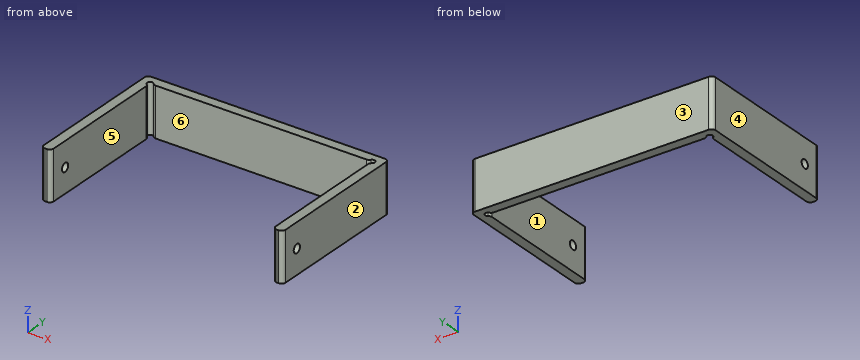
```python
from build123d import *

# Parameters (mm, degrees)
EXTRUDE_1_DEPTH     = 25
SKETCH_2_R          = 2.2
CUT_EXTRUDE_2_DEPTH = 147.215594244
SKETCH_3_R          = 1.5
CUT_EXTRUDE_3_DEPTH = 147.215594244
FILLET_1_R          = 2


with BuildPart() as part:
    # ｽｹｯﾁ1 → ﾎﾞｽ - 押し出し1 (new body)
    with BuildSketch(Plane.XY):
        Polygon((0, 0), (0, 75), (123, 75), (123, 0), (118, 0), (118, 70), (5, 70), (5, 0), align=None)
    extrude(amount=EXTRUDE_1_DEPTH)

    # ｽｹｯﾁ2 → ｶｯﾄ - 押し出し2 (cut, through all)
    with BuildSketch(Plane(origin=(123, 0, 0), x_dir=(0, 0, -1), z_dir=(1, 0, 0))):
        with Locations((-12.5, 10)):
            Circle(SKETCH_2_R)
    extrude(amount=-CUT_EXTRUDE_2_DEPTH, mode=Mode.SUBTRACT)

    # ｽｹｯﾁ3 → ｶｯﾄ - 押し出し3 (cut, through all)
    with BuildSketch(Plane.XY.offset(25)):
        with Locations((5, 70)):
            Circle(SKETCH_3_R)
        with Locations((118, 70)):
            Circle(SKETCH_3_R)
    extrude(amount=-CUT_EXTRUDE_3_DEPTH, mode=Mode.SUBTRACT)

    # ﾌｨﾚｯﾄ1
    fillet_1_edges = [part.edges().sort_by_distance(p)[0] for p in [
        (0, 0, 12.5),
        (0, 75, 12.5),
        (123, 75, 12.5),
        (123, 0, 12.5),
        (118, 0, 12.5),
        (5, 0, 12.5),
        (5, 68.5, 12.5),
        (6.5, 70, 12.5),
        (116.5, 70, 12.5),
        (118, 68.5, 12.5),
    ]]
    fillet(fillet_1_edges, radius=FILLET_1_R)


solid = part.part
```
Can you work these out from the model? Positions are in its coordinate system, mm. Face numbers are marked on the shaded views. A direction names the side the tool comes from. Coordinates: 2 decimals unless noted, no trailing zeros. Order: outer loops, then holes, each group sorted by start corner. A loop starts at its lowest first (then second) coordinate and runs counter-clockwise, first axis right, second up. Notation, with made-up numbers: (29, 8) -> (64, 8) arc R22 ccw to (64, 47) -> close; hole circle Ø4 at (-25, -12.75). An arc over 180 degrees is marked (long way). Write each question's results on one line, items separated by ' | '.
Item 1: I want a section at D-D, the plane x = 73.5. Write out the boundary of the cut face in (y, z), then the cut area to 3 significant figures.
Results are:
outline: (70, 0) -> (75, 0) -> (75, 25) -> (70, 25) -> close | area: 125 mm²
Item 2: Which directions (+Z, -Z, +X, -X, +Y, -Y) give clear straight access to the entire face, cutting with the end or side of a thin tool? Please do the marked faces 1 and 2.
Results are:
face 1: +Z, -Z, -Y | face 2: +Z, -Z, +X, +Y, -Y
Item 3: I want a section at A-A, the plane y = 10. Write out the boundary of the cut face in (x, z).
Results are:
outline: (0, 0) -> (5, 0) -> (5, 10.3) -> (0, 10.3) -> close; (0, 14.7) -> (5, 14.7) -> (5, 25) -> (0, 25) -> close; (118, 0) -> (123, 0) -> (123, 10.3) -> (118, 10.3) -> close; (118, 14.7) -> (123, 14.7) -> (123, 25) -> (118, 25) -> close
Item 4: If I drill on line 1 along X through (y, z) = (46, 23.5); line 2 along Y through (x, z) = (119.9, 12.5); line 3 along Y through (x, z) = (32, 14), over which ranges is the centre line in solid material (lowest first)?
Results are:
line 1: 0 to 5, 118 to 123 | line 2: 0 to 7.8, 12.2 to 75 | line 3: 70 to 75
Item 5: I want a section at B-B, the plane z = 12.5. Write out the boundary of the cut face in (x, y), then the cut area to 3 significant figures.
Results are:
outline: (0, 2) arc R2 ccw to (2, 0) -> (3, 0) arc R2 ccw to (5, 2) -> (5, 7.8) -> (0, 7.8) -> close; (0, 12.2) -> (5, 12.2) -> (5, 67.13) arc R2 ccw to (4.14, 68.77) arc R1.5 cw (long way) to (6.23, 70.86) arc R2 ccw to (7.87, 70) -> (115.13, 70) arc R2 ccw to (116.77, 70.86) arc R1.5 cw (long way) to (118.86, 68.77) arc R2 ccw to (118, 67.13) -> (118, 12.2) -> (123, 12.2) -> (123, 73) arc R2 ccw to (121, 75) -> (2, 75) arc R2 ccw to (0, 73) -> close; (118, 2) arc R2 ccw to (120, 0) -> (121, 0) arc R2 ccw to (123, 2) -> (123, 7.8) -> (118, 7.8) -> close | area: 1,250 mm²
Item 6: If we mould it in two halves opening along X, with no side actions, what happens to the marked faces 3, 4, 5 and 6? For each: +X half, -X half, draft (parallel to the pull), parting line (faces both ways), or undercut.
Results are:
face 3: draft | face 4: -X half | face 5: undercut | face 6: undercut
Item 7: I'm going to push a flat-ended pin straight in: pin 1 Ø12 at (x, z) = (86, 15) entering from -Y. Where does the tip first touch, or does it pass through?
Results are:
pin 1: y = 70
Item 8: I want a section at C-C, the plane y = 30. Write out the boundary of the cut face in (x, z).
Results are:
outline: (0, 0) -> (5, 0) -> (5, 25) -> (0, 25) -> close; (118, 0) -> (123, 0) -> (123, 25) -> (118, 25) -> close
